```python
from build123d import *

# Parameters (mm, degrees)
SKETCH1_R           = 2.5
BOSS_EXTRUDE1_DEPTH = 189.096108091
SCALE_2_SCALE       = 3
SCALE_3_SCALE       = 6
SCALE_5_SCALE       = 2
SCALE_6_SCALE       = 0.25
SCALE_7_SCALE       = 0.125
SCALE_8_SCALE       = 0.25
SCALE_9_SCALE       = 4
SCALE_10_SCALE      = 4
OTHER_START         = -17.55
OTHER_1_OUTLINE_R   = 5
OTHER_1_DEPTH       = 10


# Read off the part's stored shape, not the designer's step: 孔1
with BuildPart() as part:
    # Sketch1 → Boss-Extrude1 (new body)
    with BuildSketch(Plane.XY):
        with BuildLine():
            Line((2.839339828, 3.9), (5.5, 6.560660172))
            Line((5.5, 6.560660172), (5.5, 8.2))
            Line((5.5, 8.2), (3.1, 8.2))
            Line((3.1, 8.2), (3.1, 9.5))
            Line((3.1, 9.5), (3.6, 9.5))
            Line((3.6, 9.5), (3.6, 10))
            Line((3.6, 10), (8.5, 10))
            ThreePointArc((8.5, 10), (9.560660172, 9.560660172), (10, 8.5))
            Line((10, 8.5), (10, 3.6))
            Line((10, 3.6), (9.5, 3.6))
            Line((9.5, 3.6), (9.5, 3.1))
            Line((9.5, 3.1), (8.2, 3.1))
            Line((8.2, 3.1), (8.2, 5.5))
            Line((8.2, 5.5), (6.560660172, 5.5))
            Line((6.560660172, 5.5), (3.9, 2.839339828))
            Line((3.9, 2.839339828), (3.9, -2.839339828))
            Line((3.9, -2.839339828), (6.560660172, -5.5))
            Line((6.560660172, -5.5), (8.2, -5.5))
            Line((8.2, -5.5), (8.2, -3.1))
            Line((8.2, -3.1), (9.5, -3.1))
            Line((9.5, -3.1), (9.5, -3.6))
            Line((9.5, -3.6), (10, -3.6))
            Line((10, -3.6), (10, -8.5))
            ThreePointArc((10, -8.5), (9.560660172, -9.560660172), (8.5, -10))
            Line((8.5, -10), (3.6, -10))
            Line((3.6, -10), (3.6, -9.5))
            Line((3.6, -9.5), (3.1, -9.5))
            Line((3.1, -9.5), (3.1, -8.2))
            Line((3.1, -8.2), (5.5, -8.2))
            Line((5.5, -8.2), (5.5, -6.560660172))
            Line((5.5, -6.560660172), (2.839339828, -3.9))
            Line((2.839339828, -3.9), (-2.839339828, -3.9))
            Line((-2.839339828, -3.9), (-5.5, -6.560660172))
            Line((-5.5, -6.560660172), (-5.5, -8.2))
            Line((-5.5, -8.2), (-3.1, -8.2))
            Line((-3.1, -8.2), (-3.1, -9.5))
            Line((-3.1, -9.5), (-3.6, -9.5))
            Line((-3.6, -9.5), (-3.6, -10))
            Line((-3.6, -10), (-8.5, -10))
            ThreePointArc((-8.5, -10), (-9.560660172, -9.560660172), (-10, -8.5))
            Line((-10, -8.5), (-10, -3.6))
            Line((-10, -3.6), (-9.5, -3.6))
            Line((-9.5, -3.6), (-9.5, -3.1))
            Line((-9.5, -3.1), (-8.2, -3.1))
            Line((-8.2, -3.1), (-8.2, -5.5))
            Line((-8.2, -5.5), (-6.560660172, -5.5))
            Line((-6.560660172, -5.5), (-3.9, -2.839339828))
            Line((-3.9, -2.839339828), (-3.9, 2.839339828))
            Line((-3.9, 2.839339828), (-6.560660172, 5.5))
            Line((-6.560660172, 5.5), (-8.2, 5.5))
            Line((-8.2, 5.5), (-8.2, 3.1))
            Line((-8.2, 3.1), (-9.5, 3.1))
            Line((-9.5, 3.1), (-9.5, 3.6))
            Line((-9.5, 3.6), (-10, 3.6))
            Line((-10, 3.6), (-10, 8.5))
            ThreePointArc((-10, 8.5), (-9.560660172, 9.560660172), (-8.5, 10))
            Line((-8.5, 10), (-3.6, 10))
            Line((-3.6, 10), (-3.6, 9.5))
            Line((-3.6, 9.5), (-3.1, 9.5))
            Line((-3.1, 9.5), (-3.1, 8.2))
            Line((-3.1, 8.2), (-5.5, 8.2))
            Line((-5.5, 8.2), (-5.5, 6.560660172))
            Line((-5.5, 6.560660172), (-2.839339828, 3.9))
            Line((-2.839339828, 3.9), (2.839339828, 3.9))
        make_face()
        with Locations((0, 0.235847297)):
            Circle(SKETCH1_R, mode=Mode.SUBTRACT)
    extrude(amount=BOSS_EXTRUDE1_DEPTH)


with BuildPart() as part_1:
    # 缩放比例2: scaled about (0, -0.027095247, 94.548054046)
    add(part.part.scale(SCALE_2_SCALE).moved(Location((0, 0.054190494, -189.096108092))))


with BuildPart() as part_2:
    # 缩放比例3: scaled about (0, -0.027095247, 94.548054045)
    add(part_1.part.scale(SCALE_3_SCALE).moved(Location((0, 0.135476235, -472.740270225))))


with BuildPart() as part_3:
    # 缩放比例5: scaled about (0, -0.027095249, 94.548054043)
    add(part_2.part.scale(SCALE_5_SCALE).moved(Location((0, 0.027095249, -94.548054043))))


with BuildPart() as part_4:
    # 缩放比例6: scaled about (0, -0.027095249, 94.548054044)
    add(part_3.part.scale(SCALE_6_SCALE).moved(Location((0, -0.020321437, 70.911040533))))


with BuildPart() as part_5:
    # 缩放比例7: scaled about (0, -0.027095249, 94.548054044)
    add(part_4.part.scale(SCALE_7_SCALE).moved(Location((0, -0.023708343, 82.729547289))))


with BuildPart() as part_6:
    # 缩放比例8: scaled about (0, -0.027095249, 94.548054044)
    add(part_5.part.scale(SCALE_8_SCALE).moved(Location((0, -0.020321437, 70.911040533))))


with BuildPart() as part_7:
    # 缩放比例9: scaled about (0, -0.027095249, 94.548054044)
    add(part_6.part.scale(SCALE_9_SCALE).moved(Location((0, 0.081285747, -283.644162132))))


with BuildPart() as part_8:
    # 缩放比例10: scaled about (0, -0.027095249, 94.548054044)
    add(part_7.part.scale(SCALE_10_SCALE).moved(Location((0, 0.081285747, -283.644162132))))

    # 孔1 outline → 孔1 (cut)
    with BuildSketch(Plane.YZ.offset(OTHER_START)):
        with Locations((7.344833538, 1.297306883)):
            Circle(OTHER_1_OUTLINE_R)
    extrude(amount=OTHER_1_DEPTH, mode=Mode.SUBTRACT)


solid = part_8.part
```
CAD build for the part. Positions are in the model's coordinates, mm. A direction names the side the tool comes from. Coordinates: 2 decimals unless noted, no trailing zeros. Loops run counter-clockwise (first coordinate to the right, second up) from the corner with the lowest first, then second, coordinate; pieces in that order, holes last. Notation, with made-up numbers: (73.5, 31.5) - (125.5, 31.5) arc R18 ccw to (125.5, 52.5) - close; hole circle Ø5 at (5.25, 8). An arc over 180 degrees is marked (long way). Use CSV: the item, a comma, the result in double quotes. Start each with the question number.
Q1. Drop flat-ended pins along their axis: P1, Ø3, axis at y = 10.5, z = 1.5, coming from the -X side; P2, Ø2.5, axis at x = 44.5, z = 269.5, coming from the -Y side; P3, Ø0.7, axis at y = -43.5, z = -2.5, coming from the -X side. Give the stop position or say it passes through.
Q2. Probe probe 1 along X at (y, z) = (0, -31.5); probe 2 along X at (y, z) = (19.5, 316); probe 3 along Y at (x, z) = (-1, 157). List the from-to ranges inside material, lowest first. Write a range as from..to.
Q3. Cut at A-A, the plane x = 0. List the corners of the cut face in (y, z).
Q4. Two-plate mould, pull along Y, no slides. Class faces 1 (the flat face through (-27, -44.905, 89)), 2 (the flat face through (45, 27, 89)), 3 (the flat face through (17.55, 0, 89)), 4 (the cylindrical face through (6.05, 10.64, 88.59)): +Y half, -Y half, draft (parallel to the pull), parting line (faces both ways), or undercut.
Q5. 3-axis set-ups, long thin cutter, end or side, ignore diameter. For faces 5 (the flat face through (0, 17.645, 89)), 6 (the flat face through (-45, -27, 89)), 7 (the flat face through (27, 45.095, 89)), 8 (the flat face through (0, -17.455, 89)), 9 (the flat face through (-17.55, 0, 89)): which of +Z, -Z, +X, -X, +Y, -Y reach the whole face in a straight line?
Here are the results:
1,P1,"x = -7.55"
1,P2,"y = -42.69"
1,P3,"x = -42.79"
2,probe 1,"-17.55..-11.19, 11.19..17.55"
2,probe 2,"-45..-36.9, -24.18..-14.63, 14.63..24.18, 36.9..45"
2,probe 3,"-17.46..-10.05, 12.36..17.64"
3,outline,"(-17.46, -330.92) - (-10.09, -330.92) - (-10.09, 520.01) - (-17.46, 520.01) - close; (12.41, -330.92) - (17.64, -330.92) - (17.64, 520.01) - (12.41, 520.01) - close"
4,face 1,"-Y half"
4,face 2,"draft"
4,face 3,"undercut"
4,face 4,"undercut"
5,face 5,"+Z, -Z, +Y"
5,face 6,"+Z, -Z, -X, +Y, -Y"
5,face 7,"+Z, -Z, +X, -X, +Y"
5,face 8,"+Z, -Z, -Y"
5,face 9,"+Z, -Z, -X"
